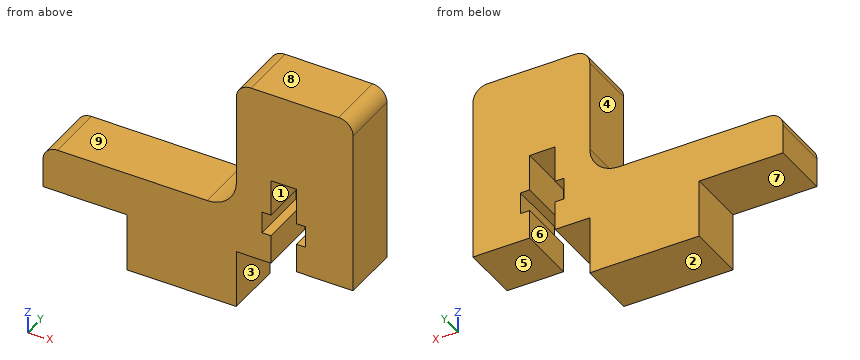
Autodesk Inventor part; units mm, degrees
ref_plane "Work Plane1" through (0, 4, 0) normal (0, 1, 0) x (-1, 0, 0)
ref_plane "Work Plane2" through (-9.5, 0, -12.5) normal (1, 0, 0) x (0, 0, -1)
ref_plane "YZ Plane" through (0, 0, 0) normal (1, 0, 0) x (0, 1, 0)
sketch "Sketch1" plane through (0, 0, 0) normal (0, 1, 0) x (-1, 0, 0)
  line L0 (0, 0) -> (16, 0)
  line L1 (16, 0) -> (16, -18.5)
  line L2 (0, -24.5) -> (0, 0)
  line L3 (0, -24.5) -> (16, -24.5)
  line L4 (11.25, -24.5) -> (11.25, -20.5)
  line L5 (11.25, -20.5) -> (12.5, -20.5)
  line L6 (12.5, -20.5) -> (12.5, -17.5)
  line L7 (12.5, -17.5) -> (11.25, -17.5)
  line L8 (11.25, -17.5) -> (11.25, -12.5)
  line L9 (11.25, -12.5) -> (7.75, -12.5)
  line L10 (7.75, -12.5) -> (7.75, -17.5)
  line L11 (7.75, -17.5) -> (6.5, -17.5)
  line L12 (6.5, -17.5) -> (6.5, -20.5)
  line L13 (6.5, -20.5) -> (7.75, -20.5)
  line L14 (7.75, -24.5) -> (7.75, -20.5)
  line L15 (16, -18.5) -> (42.5, -18.5)
  line L16 (42.5, -18.5) -> (42.5, -24.5)
  line L17 (42.5, -24.5) -> (31, -24.5)
  line L18 (31, -24.5) -> (31, -32.5)
  line L19 (31, -32.5) -> (16, -32.5)
  line L20 (16, -32.5) -> (16, -24.5)
  line L21 (9.5, -12.5) -> (9.5, -24.5) construction
  dimension "d0" = 24.5
  dimension "d1" = 16
  dimension "d4" = 3.5
  dimension "d5" = 6
  dimension "d6" = 4
  dimension "d7" = 3
  dimension "d8" = 5
  dimension "d23" = 7.75
  dimension "d24" = 6
  dimension "d25" = 14
  dimension "d26" = 42.5
  dimension "d27" = 11.5
  dimension "d28" = 15
  dimension "d29" = 32.5
extrude "Extrusion1" add sketch "Sketch1" along normal blind 8 contours L0 L1 L15 L16 L17 L18 L19 L20 L3 L4 L5 L6 L7 L8 L9 L10 L11 L12 L13 L14 L2
fillet "Fillet1" radius 2 3 edges at (-16, 4, 0) (0, 4, 0) (-42.5, 4, -18.5)
fillet "Fillet2" radius 4 1 edges at (-16, 4, -18.5)
ref_plane "Work Plane1" through (0, 4, 0) normal (0, 1, 0) x (-1, 0, 0)
ref_plane "Work Plane2" through (-9.5, 0, -12.5) normal (1, 0, 0) x (0, 0, -1)
equation "\"d31\" = 0.5 * THICKNESS"
properties part number "A8-0017"
Build history of the part. All positions in model axes, mm. Face numbers are marked on the shaded views. A direction names the side the tool comes from. Give positions to 0.01 mm unless a question says otherwise; leave off trailing zeros. Order: outer loops, then holes, each group sorted by start corner. A loop starts at its lowest first (then second) coordinate and runs counter-clockwise, first axis right, second up. Notation, with made-up numbers: M 2,54.5 L 51,54.5 A20 ccw 51,82.5 Z; hole C 27.5,6.25 d10. An arc over 180 degrees is marked long. Use one line per item in the form item = value.
1) Tool access for the marked faces 5, 6, 7, 8 and 9: list every direction of +Z, -Z, +X, -X, +Y, -Y with a clear straight run to the whole face (end or side of a thin tool).
Calculated:
face_5 = -Z, +X, +Y, -Y
face_6 = -Z, +Y, -Y
face_7 = -Z, -X, +Y, -Y
face_8 = +Z, +X, -X, +Y, -Y
face_9 = +Z, -X, +Y, -Y
2) Two-plate mould, pull along X, no slides. Class the marked faces 1, 2, 3 and 4: released by +X, released by -X, zero draft, split by the parting line, or undercut.
Calculated:
face_1 = undercut
face_2 = zero draft
face_3 = released by +X
face_4 = released by -X
3) Saw through at C-C (x = -23.5). Give the cut face in (y, z).
Calculated:
outline = M 0,-32.5 L 8,-32.5 L 8,-18.5 L 0,-18.5 Z
4) Saw through at B-B (y = 3.5). Give the cut face in (x, z).
Calculated:
outline = M -42.5,-24.5 L -31,-24.5 L -31,-32.5 L -16,-32.5 L -16,-24.5 L -11.25,-24.5 L -11.25,-20.5 L -12.5,-20.5 L -12.5,-17.5 L -11.25,-17.5 L -11.25,-12.5 L -7.75,-12.5 L -7.75,-17.5 L -6.5,-17.5 L -6.5,-20.5 L -7.75,-20.5 L -7.75,-24.5 L 0,-24.5 L 0,-2 A2 ccw -2,0 L -14,0 A2 ccw -16,-2 L -16,-14.5 A4 cw -20,-18.5 L -40.5,-18.5 A2 ccw -42.5,-20.5 Z
5) Saw through at D-D (z = -29). Give the cut face in (x, y).
Calculated:
outline = M -31,0 L -16,0 L -16,8 L -31,8 Z
6) Saw through at A-A (z = -21). Give the cut face in (x, y), plus the area to 3 significant figures.
Calculated:
outline = M -42.5,0 L -11.25,0 L -11.25,8 L -42.5,8 Z; M -7.75,0 L 0,0 L 0,8 L -7.75,8 Z
area = 312 mm2
7) Probe probe 1 along X at (y, z) = (2.75, -22); probe 2 along X at (y, z) = (4.75, -14); probe 3 along Z at (x, y) = (-11, 7.5). List the from-to ranges inside material, lowest first.
Calculated:
probe_1 = -42.5 to -11.25, -7.75 to 0
probe_2 = -16 to -11.25, -7.75 to 0
probe_3 = -12.5 to 0
8) Drop flat-ended pins along their axis: pin 1 (1.5 mm diameter, centred on y = 5.5, z = -14, fed in from -X); pin 2 (2.5 mm diameter, centred on y = 6, z = -15, fed in from +X); pin 3 (2.5 mm diameter, centred on y = 4.5, z = -15.5, fed in from -X); pin 4 (4 mm diameter, centred on x = -2.5, y = 4, fed in from -Z). Give the stop position or say it passes through.
Calculated:
pin_1 = -16.01
pin_2 = 0
pin_3 = -16.69
pin_4 = -24.5
